from build123d import *

# Parameters (mm, degrees)
SKETCH1_W                    = 500
SKETCH1_H                    = 574
BOSS_EXTRUDE1_DEPTH          = 2
CONVERT_SOLID1_OUTLINE_W     = 500
CONVERT_SOLID1_OUTLINE_H     = 574
CONVERT_SOLID1_DEPTH         = 1
EDGE_FLANGE1_STRIP_W         = 6
EDGE_FLANGE1_STRIP_H         = 1
EDGE_FLANGE1_STRIP_CUT_DEPTH = 574
EDGE_FLANGE1_DEPTH           = 574
SKETCH11_W                   = 280
SKETCH11_H                   = 472
CUT_EXTRUDE1_DEPTH           = 600
SKETCH12_R                   = 50.5
CUT_EXTRUDE2_DEPTH           = 10
SKETCH13_R                   = 6
CUT_EXTRUDE3_DEPTH           = 12
FILLET2_R                    = 2
CUT_EXTRUDE7_START           = -499
CUT_EXTRUDE7_OUTLINE_R       = 3.55
CUT_EXTRUDE7_DEPTH           = 502


# Read off the part's stored shape, not the designer's step: Convert-Solid1, Cut-Extrude7
# Sheet-metal steps are written as plain solids
with BuildPart() as part:
    # Sketch1 → Boss-Extrude1 (new body)
    with BuildSketch(Plane(origin=(0, 0, 0), x_dir=(1, 0, 0), z_dir=(0, 1, 0))):
        Rectangle(SKETCH1_W, SKETCH1_H)
    extrude(amount=BOSS_EXTRUDE1_DEPTH)

    # Convert-Solid1 outline → Convert-Solid1 (cut)
    with BuildSketch(Plane(origin=(0, 0, 0), x_dir=(1, 0, 0), z_dir=(0, 1, 0))):
        Rectangle(CONVERT_SOLID1_OUTLINE_W, CONVERT_SOLID1_OUTLINE_H)
    extrude(amount=CONVERT_SOLID1_DEPTH, mode=Mode.SUBTRACT)

    # Edge-Flange1 strip (across the edge) → Edge-Flange1 strip cut (cut)
    with BuildSketch(Plane(origin=(-250, 1, 287), x_dir=(1, 0, 0), z_dir=(0, 0, -1))):
        with Locations((-2, -0.5)):
            Rectangle(EDGE_FLANGE1_STRIP_W, EDGE_FLANGE1_STRIP_H)
    edge_flange1_strip_cut = extrude(amount=EDGE_FLANGE1_STRIP_CUT_DEPTH, mode=Mode.SUBTRACT)

    # Edge-Flange1 section (across the edge) → Edge-Flange1 (add)
    with BuildSketch(Plane(origin=(-250, 1, 287), x_dir=(1, 0, 0), z_dir=(0, 0, -1))):
        with BuildLine():
            Line((-1, 1), (-1, 945))
            Line((-1, 945), (0, 945))
            Line((0, 945), (0, 1))
            ThreePointArc((0, 1), (0.292893219, 0.292893219), (1, 0))
            Line((1, 0), (1, -1))
            ThreePointArc((1, -1), (-0.414213562, -0.414213562), (-1, 1))
        make_face()
    edge_flange1 = extrude(amount=EDGE_FLANGE1_DEPTH)

    # Mirror1: Edge-Flange1 strip cut, Edge-Flange1 across plane
    add(edge_flange1_strip_cut.mirror(Plane(origin=(0, 0, 0), x_dir=(0, 0, 1), z_dir=(1, 0, 0))), mode=Mode.SUBTRACT)
    add(edge_flange1.mirror(Plane(origin=(0, 0, 0), x_dir=(0, 0, 1), z_dir=(1, 0, 0))))

    # Sketch11 → Cut-Extrude1 (cut)
    with BuildSketch(Plane(origin=(251, 40.165636604, 898.471308301), x_dir=(0, 1, 0), z_dir=(1, 0, 0))):
        with Locations((-624.165636604, -898.471308301)):
            Rectangle(SKETCH11_W, SKETCH11_H)
        with BuildLine():
            Line((-189.165636604, -662.471308301), (-79.165636604, -662.471308301))
            ThreePointArc((-79.165636604, -662.471308301), (-72.094568792, -665.400240489), (-69.165636604, -672.471308301))
            Line((-69.165636604, -672.471308301), (-69.165636604, -1124.471308301))
            ThreePointArc((-69.165636604, -1124.471308301), (-72.094568792, -1131.542376113), (-79.165636604, -1134.471308301))
            Line((-79.165636604, -1134.471308301), (-189.165636604, -1134.471308301))
            ThreePointArc((-189.165636604, -1134.471308301), (-196.236704416, -1131.542376113), (-199.165636604, -1124.471308301))
            Line((-199.165636604, -1124.471308301), (-199.165636604, -672.471308301))
            ThreePointArc((-199.165636604, -672.471308301), (-196.236704416, -665.400240489), (-189.165636604, -662.471308301))
        make_face()
    extrude(amount=-CUT_EXTRUDE1_DEPTH, mode=Mode.SUBTRACT)

    # Sketch12 → Cut-Extrude2 (cut)
    with BuildSketch(Plane(origin=(251, 40.165636604, 898.471308301), x_dir=(0, 1, 0), z_dir=(1, 0, 0))):
        with Locations((-914.165636604, -898.471308301)):
            Circle(SKETCH12_R)
    extrude(amount=-CUT_EXTRUDE2_DEPTH, mode=Mode.SUBTRACT)

    # Sketch13 → Cut-Extrude3 (cut)
    with BuildSketch(Plane(origin=(-635.072358446, 2, 898.471308301), x_dir=(-1, 0, 0), z_dir=(0, 1, 0))):
        with Locations(Location((-804.072358446, -693.471308301, 0), (0, 0, 90))):
            Circle(SKETCH13_R)
        with Locations(Location((-466.072358446, -693.471308301, 0), (0, 0, 270))):
            Circle(SKETCH13_R)
        with Locations(Location((-466.072358446, -1103.471308301, 0), (0, 0, 90))):
            Circle(SKETCH13_R)
        with Locations(Location((-804.072358446, -1103.471308301, 0), (0, 0, 270))):
            Circle(SKETCH13_R)
    extrude(amount=-CUT_EXTRUDE3_DEPTH, mode=Mode.SUBTRACT)

    # Fillet2
    fillet2_edges = [part.edges().sort_by_distance(p)[0] for p in [
        (-250.5, -944, 287),
        (-250.5, -944, -287),
        (250.5, -944, -287),
        (250.5, -944, 287),
    ]]
    fillet(fillet2_edges, radius=FILLET2_R)

    # Cut-Extrude7 outline → Cut-Extrude7 (cut)
    with BuildSketch(Plane(origin=(-248, 561.16698045, 1244.210853702), x_dir=(0, -1, 0), z_dir=(-1, 0, 0)).offset(CUT_EXTRUDE7_START)):
        with Locations((577.16698045, -1524.210853702)):
            Circle(CUT_EXTRUDE7_OUTLINE_R)
        with Locations((877.16698045, -1524.210853702)):
            Circle(CUT_EXTRUDE7_OUTLINE_R)
        with Locations((1177.16698045, -1524.210853702)):
            Circle(CUT_EXTRUDE7_OUTLINE_R)
        with Locations((1477.16698045, -1524.210853702)):
            Circle(CUT_EXTRUDE7_OUTLINE_R)
        with Locations((1498.16698045, -1244.210853702)):
            Circle(CUT_EXTRUDE7_OUTLINE_R)
        with Locations((1477.16698045, -964.210853702)):
            Circle(CUT_EXTRUDE7_OUTLINE_R)
        with Locations((1177.16698045, -964.210853702)):
            Circle(CUT_EXTRUDE7_OUTLINE_R)
        with Locations((877.16698045, -964.210853702)):
            Circle(CUT_EXTRUDE7_OUTLINE_R)
        with Locations((577.16698045, -964.210853702)):
            Circle(CUT_EXTRUDE7_OUTLINE_R)
    extrude(amount=CUT_EXTRUDE7_DEPTH, mode=Mode.SUBTRACT)


solid = part.part
Design review of the part built by this model. Coordinates are the model's own, in mm. A direction names the side the tool comes from. Coordinates: 2 decimals unless noted, no trailing zeros. Order: outer loops, then holes, each group sorted by start corner. A loop starts at its lowest first (then second) coordinate and runs counter-clockwise, first axis right, second up. Notation, with made-up numbers: M 61,66 L 120,66 A28 ccw 120,100 Z; hole C 77.25,-36.5 d11. An arc over 180 degrees is marked long. Use a Markdown table: item, result.
(1) Draft analysis for pull direction X (two halves, no side actions). For faces 1 (the cylindrical face through (250.507, -825.832, 15.169)), 2 (the flat face through (-251, -361, 4)), 3 (the flat face through (250, -374, 4)), state which applies: released by +X, released by -X, zero draft, split by the parting line, or undercut.
Worked answers:
| item | result |
|---|---|
| face 1 | zero draft |
| face 2 | released by -X |
| face 3 | undercut |
(2) Add section D-D (y = -765). Give the boundary of the cut face in (x, z).
Worked answers:
| item | result |
|---|---|
| outline | M -251,-287 L -250,-287 L -250,287 L -251,287 Z; M 250,-287 L 251,-287 L 251,287 L 250,287 Z |
(3) Add section B-B (z = -88). Give the boundary of the cut face in (x, y).
Worked answers:
| item | result |
|---|---|
| outline | M -251,-944 L -250,-944 L -250,-724 L -251,-724 Z; M -251,-444 L -250,-444 L -250,-159 L -251,-159 Z; M -251,-29 L -250,-29 L -250,0 A1 cw -249,1 L 249,1 A1 cw 250,0 L 250,-29 L 251,-29 L 251,0 A2 ccw 249,2 L -249,2 A2 ccw -251,0 Z; M 250,-944 L 251,-944 L 251,-724 L 250,-724 Z; M 250,-444 L 251,-444 L 251,-159 L 250,-159 Z |
(4) Add section C-C (y = -874). Give the boundary of the cut face in (x, z).
Worked answers:
| item | result |
|---|---|
| outline | M -251,-287 L -250,-287 L -250,287 L -251,287 Z; M 250,-287 L 251,-287 L 251,-50.5 L 250,-50.5 Z; M 250,50.5 L 251,50.5 L 251,287 L 250,287 Z |
(5) For faces 4 (the flat face through (-250, -374, 4)), 5 (the flat face through (251, -361, 4)), list the 3-axis set-ups (+Z, -Z, +X, -X, +Y, -Y) from which the entire face can be reached by the end or side of a thin tool; tool diameter is ignored.
Worked answers:
| item | result |
|---|---|
| face 4 | +Z, -Z, -Y |
| face 5 | +Z, -Z, +X, +Y, -Y |
(6) Add section A-A (y = -507). Give the boundary of the cut face in (x, z).
Worked answers:
| item | result |
|---|---|
| outline | M -251,-287 L -250,-287 L -250,-236 L -251,-236 Z; M -251,236 L -250,236 L -250,287 L -251,287 Z; M 250,-287 L 251,-287 L 251,-236 L 250,-236 Z; M 250,236 L 251,236 L 251,287 L 250,287 Z |
(7) For P1, Ø11.5, axis at y = -616, z = -280, coming from the +X side; P2, Ø12, axis at x = -171, z = -96, coming from the -Y side; P3, Ø1.1, axis at x = -250.5, z = 34.5, coming from the +Y side, all flat-tipped, find the tip position at first contact; note any pin that passes through.
Worked answers:
| item | result |
|---|---|
| P1 | stops at x = 251 |
| P2 | stops at y = 1 |
| P3 | stops at y = 1.76 |
(8) Wall thickness on probe 1 along Y at (x, z) = (250.7, 280); probe 2 along Z at (x, y) = (-250.7, -316); probe 3 along X at (y, z) = (-496.5, -242.5): over which ranges is each line inside the solid? List them lowest first.
Worked answers:
| item | result |
|---|---|
| probe 1 | y = -944 to -919.55, -912.45 to -619.55, -612.45 to -319.55, -312.45 to -19.55, -12.45 to 1.05 |
| probe 2 | z = -287 to -283.55, -276.45 to 276.45, 283.55 to 287 |
| probe 3 | x = -251 to -250, 250 to 251 |
